```python
from build123d import *

# Parameters (mm, degrees)
SKETCH1_W           = 53.34
SKETCH1_H           = 27.94
BOSS_EXTRUDE1_DEPTH = 1.524
SKETCH2_R           = 1.0922
CUT_EXTRUDE1_DEPTH  = 1.524


with BuildPart() as part:
    # Sketch1 → Boss-Extrude1 (new body)
    with BuildSketch(Plane(origin=(0, 0, 0), x_dir=(1, 0, 0), z_dir=(0, 1, 0))):
        with Locations((26.67, 13.97)):
            Rectangle(SKETCH1_W, SKETCH1_H)
    extrude(amount=BOSS_EXTRUDE1_DEPTH)

    # Sketch2 → Cut-Extrude1 (cut)
    with BuildSketch(Plane(origin=(0, 1.524, 0), x_dir=(1, 0, 0), z_dir=(0, 1, 0))):
        with Locations(Location((2.54, 25.4, 0), (0, 0, 270))):
            Circle(SKETCH2_R)
        with Locations(Location((50.8, 25.4, 0), (0, 0, 270))):
            Circle(SKETCH2_R)
        with Locations(Location((50.8, 2.54, 0), (0, 0, 270))):
            Circle(SKETCH2_R)
    extrude(amount=-CUT_EXTRUDE1_DEPTH, mode=Mode.SUBTRACT)


solid = part.part
```
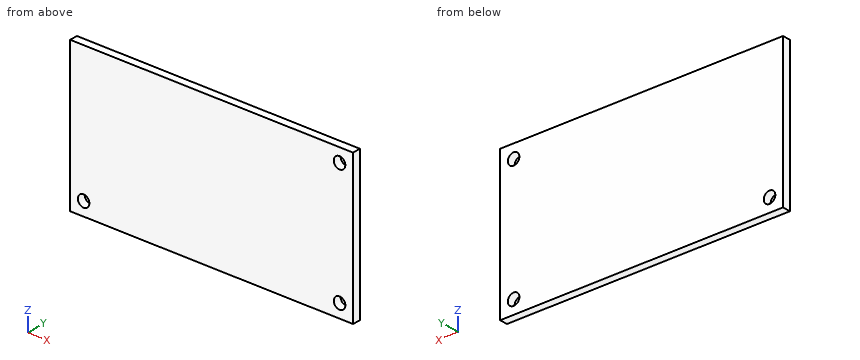
Geometry check sheet. Reference: the model listing, model coordinates, mm. Coordinates: 2 decimals unless noted, no trailing zeros. Write each loop counter-clockwise with the first axis right and the second up, starting at its lowest first coordinate (ties: lowest second). Pieces come first, ordered by that corner, then holes. Notation, with made-up numbers: (-34, 88) -> (23, 88) arc R23 cw to (23, 118) -> close; hole circle Ø5 at (7, 45.25). An arc over 180 degrees is marked (long way). Use CSV: the item, a comma, the result in double quotes. Start each with the question number.
Item 1: Cross-section at B-B, the plane x = 2.54. Record the cut outline in (y, z).
Item 2: Cross-section at A-A, the plane z = -2.54. Record the cut outline in (x, y), plus the area to 3 significant figures.
Item 3: Cross-section at C-C, the plane x = 50.8. Record the cut outline in (y, z), plus the area to 3 significant figures.
Item 4: Thickness scan on line 1 (X direction, y = 0.6, z = -25.4); line 2 (X direction, y = 0.1, z = -2.5); line 3 (Z direction, x = 51, y = 1.15). Record the ranges inside material, lowest first.
Item 5: Cross-section at D-D, the plane z = -25. Record the cut outline in (x, y), plus the area to 3 significant figures.
Answers:
1,outline,"(0, -27.94) -> (1.52, -27.94) -> (1.52, -26.49) -> (0, -26.49) -> close; (0, -24.31) -> (1.52, -24.31) -> (1.52, 0) -> (0, 0) -> close"
2,outline,"(0, 0) -> (49.71, 0) -> (49.71, 1.52) -> (0, 1.52) -> close; (51.89, 0) -> (53.34, 0) -> (53.34, 1.52) -> (51.89, 1.52) -> close"
2,area,"78.0 mm^2"
3,outline,"(0, -27.94) -> (1.52, -27.94) -> (1.52, -26.49) -> (0, -26.49) -> close; (0, -24.31) -> (1.52, -24.31) -> (1.52, -3.63) -> (0, -3.63) -> close; (0, -1.45) -> (1.52, -1.45) -> (1.52, 0) -> (0, 0) -> close"
3,area,"35.9 mm^2"
4,line 1,"0 to 1.45, 3.63 to 49.71, 51.89 to 53.34"
4,line 2,"0 to 49.71, 51.89 to 53.34"
4,line 3,"-27.94 to -26.47, -24.33 to -3.61, -1.47 to 0"
5,outline,"(0, 0) -> (1.52, 0) -> (1.52, 1.52) -> (0, 1.52) -> close; (3.56, 0) -> (49.78, 0) -> (49.78, 1.52) -> (3.56, 1.52) -> close; (51.82, 0) -> (53.34, 0) -> (53.34, 1.52) -> (51.82, 1.52) -> close"
5,area,"75.1 mm^2"
